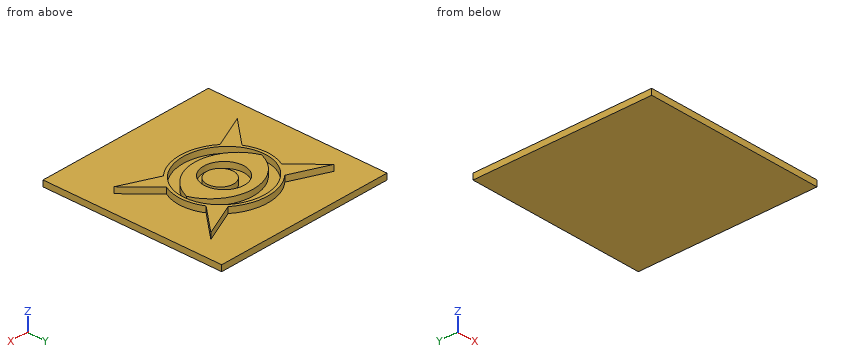
```python
from build123d import *

# Parameters (mm, degrees)
SKICA1_W                      = 300
SKICA1_H                      = 300
P_IDAT_VYSUNUT_M1_DEPTH       = 10
P_IDAT_VYSUNUT_M2_OUTLINE_R   = 34
P_IDAT_VYSUNUT_M2_OUTLINE_R_2 = 22.5
P_IDAT_VYSUNUT_M2_DEPTH       = 10


# Read off the part's stored shape, not the designer's step: Přidat vysunutím2
with BuildPart() as part:
    # Skica1 → Přidat vysunutím1 (new body)
    with BuildSketch(Plane.XY):
        with Locations((150, 150)):
            Rectangle(SKICA1_W, SKICA1_H)
    extrude(amount=P_IDAT_VYSUNUT_M1_DEPTH)

    # Přidat vysunutím2 outline → Přidat vysunutím2 (add)
    # profile 1 of 3: a face of its own
    with BuildSketch(Plane.XY.offset(10)):
        with BuildLine():
            Line((264.644345224, 249.114364816), (204.448257064, 222.313339624))
            add(Edge.make_bspline(
                [(204.448257064, 222.313339624), (153, 266.115859509), (101.551742936, 222.313339624)],
                knots=[0.839064453, 0.839064453, 0.839064453, 2.302528201, 2.302528201, 2.302528201], degree=2, weights=[1, 0.744018351, 1]))
            Line((101.551742936, 222.313339624), (41.355654776, 249.114364816))
            Line((41.355654776, 249.114364816), (84.451742425, 201.251310533))
            add(Edge.make_bspline(
                [(84.451742425, 201.251310533), (66.506189511, 168), (84.451742425, 134.748689467)],
                knots=[2.668661787, 2.668661787, 2.668661787, 3.614523521, 3.614523521, 3.614523521], degree=2, weights=[1, 0.890237111, 1]))
            Line((84.451742425, 134.748689467), (41.355654776, 86.885635184))
            Line((41.355654776, 86.885635184), (101.551742936, 113.686660376))
            add(Edge.make_bspline(
                [(101.551742936, 113.686660376), (153, 69.884140491), (204.448257064, 113.686660376)],
                knots=[3.980657106, 3.980657106, 3.980657106, 5.444120855, 5.444120855, 5.444120855], degree=2, weights=[1, 0.744018351, 1]))
            Line((204.448257064, 113.686660376), (264.644345224, 86.885635184))
            Line((264.644345224, 86.885635184), (221.548257575, 134.748689467))
            add(Edge.make_bspline(
                [(221.548257575, 134.748689467), (239.493810489, 168), (221.548257575, 201.251310533)],
                knots=[5.81025444, 5.81025444, 5.81025444, 6.756116174, 6.756116174, 6.756116174], degree=2, weights=[1, 0.890237111, 1]))
            Line((221.548257575, 201.251310533), (264.644345224, 249.114364816))
        make_face()
        with BuildLine():
            add(Edge.make_bspline(
                [(225, 168), (225, 176.864581058), (221.284259047, 194.593743175), (205.346766645, 217.22941635), (181.371826698, 232.430212202), (153, 237.784893899), (129.11147608, 233.276356498), (112.212158133, 224.593414956), (102.642030231, 216.993953421), (95.923468043, 209.682344585), (90.126433793, 201.707291075), (83.28831958, 188.170345197), (79.350635096, 167.005143483), (84.715740953, 141.406256825), (100.653233355, 118.77058365), (124.628173302, 103.569787798), (153, 98.215106101), (181.371826698, 103.569787798), (205.346766645, 118.77058365), (221.284259047, 141.406256825), (225, 159.135418942), (225, 168)],
                knots=[0, 0, 0, 0, 0.392699082, 0.785398163, 1.178097245, 1.570796327, 1.963495408, 2.170032115, 2.366381656, 2.481498811, 2.596615966, 2.792965507, 3.141592654, 3.534291735, 3.926990817, 4.319689899, 4.71238898, 5.105088062, 5.497787144, 5.890486225, 6.283185307, 6.283185307, 6.283185307, 6.283185307], degree=3))
        make_face(mode=Mode.SUBTRACT)
    # profile 2 of 3: a face of its own
    with BuildSketch(Plane.XY.offset(10)):
        with BuildLine():
            ThreePointArc((221, 168), (153, 216.5), (85, 168))
            ThreePointArc((85, 168), (153, 119.5), (221, 168))
        make_face()
        with Locations((153, 168)):
            Circle(P_IDAT_VYSUNUT_M2_OUTLINE_R, mode=Mode.SUBTRACT)
    # profile 3 of 3: a face of its own
    with BuildSketch(Plane.XY.offset(10)):
        with Locations((160, 168)):
            Circle(P_IDAT_VYSUNUT_M2_OUTLINE_R_2)
    extrude(amount=P_IDAT_VYSUNUT_M2_DEPTH)


solid = part.part
```
Check sheet for the modelled part. Datum: model origin and axes. Units: mm. Round coordinates to 2 decimals unless told otherwise and drop trailing zeros. Order: outer loops, then holes, each group sorted by start corner. A loop starts at its lowest first (then second) coordinate and runs counter-clockwise, first axis right, second up. Notation, with made-up numbers: (19.5, 89) -> (39.5, 89) arc R28 cw to (39.5, 124) -> close; hole circle Ø10 at (65.5, -13.75). An arc over 180 degrees is marked (long way). Use CSV: the item, a comma, the result in double quotes.
(1) Cross-section at A-A (z = 14). Count the separate pieces of the cut face and the enclosed holes in it, and give its area (3 significant figures).
Worked out:
separate pieces,"3"
enclosed holes,"2"
area,"13,200 mm²"
(2) Depth check by flat-ended pin: pin 1 (1 mm diameter, centred on x = 123, y = 109.5, fed in from +Z); pin 2 (4 mm diameter, centred on x = 89, z = 17.5, fed in from -Y); pin 3 (4 mm diameter, centred on x = 62.5, z = 14.5, fed in from -Y). Enter the tip coordinate at first touch or a pass-through.
Worked out:
pin 1,"z = 10"
pin 2,"y = 107.21"
pin 3,"y = 95.41"
(3) Material ranges on line 1 along Y through (x, z) = (153, 17); line 2 along X through (y, z) = (185.5, 12); line 3 along X through (y, z) = (131, 13.5), recorded low to high. Write a range as from..to.
Worked out:
line 1,"95..100, 119.5..134, 146.62..189.38, 202..216.5, 236..241"
line 2,"78.25..83.43, 93.86..123.85, 145.86..174.14, 182.15..212.14, 222.57..227.75"
line 3,"81.08..92.6, 113.99..192.01, 213.4..224.92"
(4) Cross-section at D-D (x = 251). Record the boundary of the cut face in (y, z).
Worked out:
outline,"(0, 0) -> (300, 0) -> (300, 10) -> (243.04, 10) -> (243.04, 20) -> (233.96, 20) -> (233.96, 10) -> (102.04, 10) -> (102.04, 20) -> (92.96, 20) -> (92.96, 10) -> (0, 10) -> close"
(5) Cross-section at B-B (x = 57). Record the boundary of the cut face in (y, z), and give its area (3 significant figures).
Worked out:
outline,"(0, 0) -> (300, 0) -> (300, 10) -> (242.15, 10) -> (242.15, 20) -> (231.74, 20) -> (231.74, 10) -> (104.26, 10) -> (104.26, 20) -> (93.85, 20) -> (93.85, 10) -> (0, 10) -> close"
area,"3,210 mm²"
(6) Cross-section at C-C (y = 80). Record the boundary of the cut face in (x, z), and give its area (3 significant figures).
Worked out:
outline,"(0, 0) -> (300, 0) -> (300, 10) -> (0, 10) -> close"
area,"3,000 mm²"
